Job drawing, mm, ordinate dimensions from the low corner. One solid piece. A direction names the side the tool comes from. Coordinates: 2 decimals unless noted, no trailing zeros. Order: outer loops, then holes, each group sorted by start corner. A loop starts at its lowest first (then second) coordinate and runs counter-clockwise, first axis right, second up. Notation, with made-up numbers: (59, 8) - (73, 8) arc R33 ccw to (73, 41) - close; hole circle Ø1 at (39, 87.25). An arc over 180 degrees is marked (long way). Return JSON: item names as keys, results as strings.
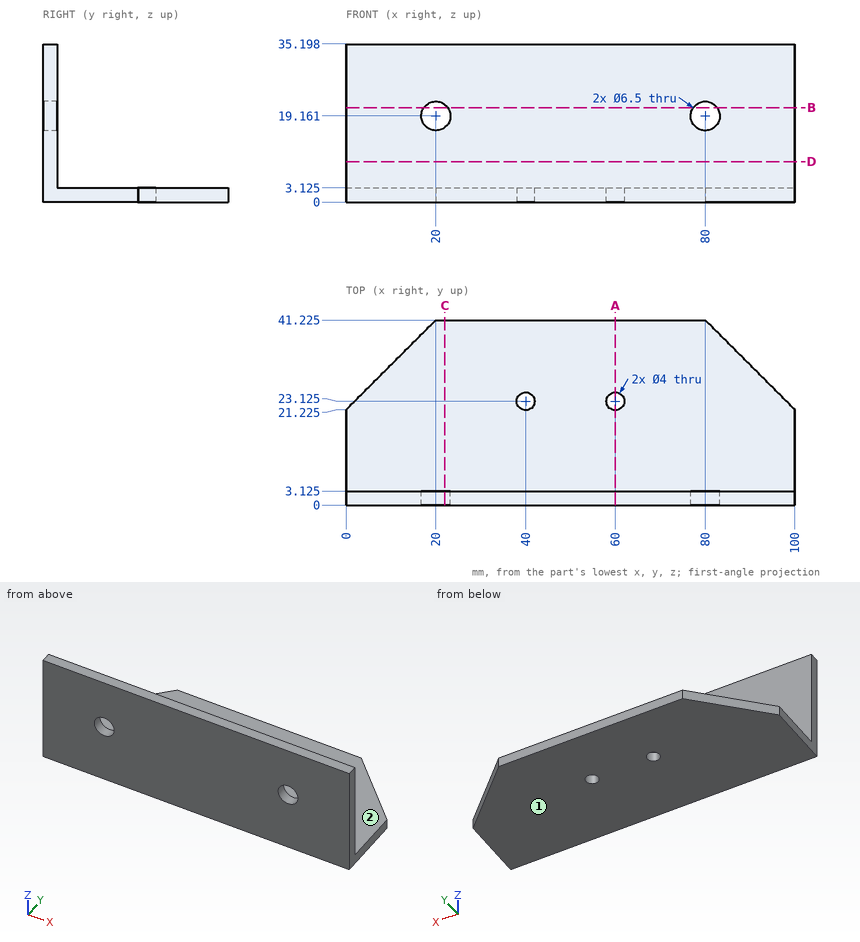
1. Tool access for the marked faces 1 and 2: list every direction of +Z, -Z, +X, -X, +Y, -Y with a clear straight run to the whole face (end or side of a thin tool).
Check values:
{"face 1": "-Z, +X, -X, +Y, -Y", "face 2": "+Z, +X, -X, +Y"}
2. Probe L1, parallel to Y at x = 40, z = 2 (1 decimal); L2, parallel to Z at x = 44.5, y = 38 (1 decimal). List the from-to ranges inside material, lowest first.
Check values:
{"L1": "0 to 21.1, 25.1 to 41.2", "L2": "0 to 3.1"}
3. Cut at C-C on x = 22. Give the cut face in (y, z) (1 decimal), plus the area to 3 significant figures.
Check values:
{"outline": "(0, 0) - (41.2, 0) - (41.2, 3.1) - (3.1, 3.1) - (3.1, 16.6) - (0, 16.6) - close; (0, 21.7) - (3.1, 21.7) - (3.1, 35.2) - (0, 35.2) - close", "area": "213 mm²"}
4. Drop flat-ended pins along their axis: pin 1 (5 mm diameter, centred on x = 74.5, z = 20.5, fed in from -Y); pin 2 (19 mm diameter, centred on x = 29.5, y = 26.5, fed in from +Z) (1 decimal); pin 3 (8.5 mm diameter, centred on x = 20, z = 19.16, fed in from +Y) (1 decimal). Give the stop position or say it passes through.
Check values:
{"pin 1": "y = 0", "pin 2": "z = 3.1", "pin 3": "y = 3.1"}
5. Cut at D-D on z = 9. Give the cut face in (x, y) (1 decimal).
Check values:
{"outline": "(0, 0) - (100, 0) - (100, 3.1) - (0, 3.1) - close"}
6. Cut at B-B on z = 21. Give the cut face in (x, y) (1 decimal), plus the area to 3 significant figures.
Check values:
{"outline": "(0, 0) - (17.3, 0) - (17.3, 3.1) - (0, 3.1) - close; (22.7, 0) - (77.3, 0) - (77.3, 3.1) - (22.7, 3.1) - close; (82.7, 0) - (100, 0) - (100, 3.1) - (82.7, 3.1) - close", "area": "279 mm²"}
7. Cut at A-A on x = 60. Give the cut face in (y, z) (1 decimal).
Check values:
{"outline": "(0, 0) - (21.1, 0) - (21.1, 3.1) - (3.1, 3.1) - (3.1, 35.2) - (0, 35.2) - close; (25.1, 0) - (41.2, 0) - (41.2, 3.1) - (25.1, 3.1) - close"}
